from build123d import *

# Parameters (mm, degrees)
SKETCH1_R                    = 4.7625
BOSS_EXTRUDE1_DEPTH          = 588.772
BOSS_EXTRUDE2_START          = 91.186
SKETCH1_3_R                  = 6.35
SKETCH1_3_R_2                = 4.7625
BOSS_EXTRUDE2_DEPTH          = 406.4
F_25_0_1495_DIAMETER_HOLE1_D = 3.7973


with BuildPart() as part:
    # Sketch1 → Boss-Extrude1 (new body)
    with BuildSketch(Plane.XY):
        Circle(SKETCH1_R)
    extrude(amount=BOSS_EXTRUDE1_DEPTH)

    # Sketch1<3> → Boss-Extrude2 (add)
    with BuildSketch(Plane.XY.offset(BOSS_EXTRUDE2_START)):
        Circle(SKETCH1_3_R)
        Circle(SKETCH1_3_R_2, mode=Mode.SUBTRACT)
    extrude(amount=BOSS_EXTRUDE2_DEPTH)

    # #25 (0.1495) Diameter Hole1 (through all)
    with Locations(Plane.XY.offset(588.772)):
        with Locations((0, 0)):
            Hole(F_25_0_1495_DIAMETER_HOLE1_D / 2)


solid = part.part
Input: part model. Units: mm. Frame: model coordinates. A direction names the side the tool comes from. Give positions to 0.01 mm unless a question says otherwise; leave off trailing zeros. Write each loop counter-clockwise with the first axis right and the second up, starting at its lowest first coordinate (ties: lowest second). Pieces come first, ordered by that corner, then holes. Notation, with made-up numbers: M -8.5,-16 L 45.5,-16 A14 cw 45.5,11 Z; hole C -37,25 d1. An arc over 180 degrees is marked long. Use one line per item in the form item = value.
1. Cut plane A-A on z = 382. Return loops of the section in (x, y), and give its area (3 significant figures).
Outcome:
outline = C 0,0 d12.7; hole C 0,0 d3.8
area = 115 mm²
2. Cut plane B-B on z = 546. Return loops of the section in (x, y) (1 decimal), and give its area (3 significant figures).
Outcome:
outline = C 0,0 d9.5; hole C 0,0 d3.8
area = 59.9 mm²
3. Ray query, L1, parallel to Y at x = 0, z = 336.5; L2, parallel to Z at x = 5.5, y = -0.75; L3, parallel to Y at x = 0.25, z = 45. Return the intervals inside material, ascending.
Outcome:
L1 = -6.35 to -1.9, 1.9 to 6.35
L2 = 91.19 to 497.59
L3 = -4.76 to -1.88, 1.88 to 4.76
4. First-contact query: P1, Ø1, axis at y = 2, z = 345, coming from the +X side; P2, Ø1.5, axis at y = 1.5, z = 485.5, coming from the -X side. Flat tips, straight axial feed; report the tip coordinate or a pass-through.
Outcome:
P1 = 6.17
P2 = -6.31
5. Reachability of faces 1 (the face through (1, 5, 91.186)), 2 (the face through (-3.78, -2.9, 542.54)), 3 (the face through (2.05, 0.07, 0)) from +Z, -Z, +X, -X, +Y, -Y: full face, straight path, thin tool, end or side. Return the list, or none.
Outcome:
face_1 = -Z
face_2 = +Z
face_3 = -Z, +X, -X, +Y, -Y
